The listing builds one solid part. Answer for the finished solid, in the listing's coordinates (mm). Give positions to 0.01 mm unless a question says otherwise; leave off trailing zeros. Write each loop counter-clockwise with the first axis right and the second up, starting at its lowest first coordinate (ties: lowest second). Pieces come first, ordered by that corner, then holes. Notation, with made-up numbers: M 81.5,69 L 100.5,69 A25 cw 100.5,108 Z; hole C 38,-37 d4. An arc over 180 degrees is marked long. Answer as a JSON object with one key per item and string values.
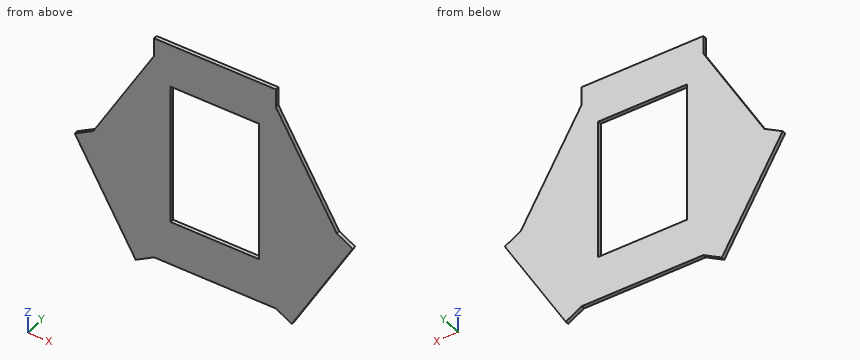
```python
from build123d import *

# Parameters (mm, degrees)
SKETCH1_W           = 120
SKETCH1_H           = 192
SKETCH1_W_2         = 165
SKETCH1_H_2         = 25
BOSS_EXTRUDE2_DEPTH = 5


with BuildPart() as part:
    # Sketch1 → Boss-Extrude2 (new body)
    with BuildSketch(Plane(origin=(0, 0, 0), x_dir=(1, 0, 0), z_dir=(0, 1, 0))):
        Polygon((-165, 0), (-82.5, -142.894191624), (82.5, -142.894191624), (165, 0), (82.5, 142.894191624), (-82.5, 142.894191624), align=None)
        with Locations((0, -13.105808376)):
            Rectangle(SKETCH1_W, SKETCH1_H, mode=Mode.SUBTRACT)
        Polygon((-82.5, 142.894191624), (-107.5, 157.327948354), (-190, 14.43375673), (-165, 0), align=None)
        Polygon((104.150635095, 155.394191624), (186.650635095, 12.5), (165, 0), (82.5, 142.894191624), align=None)
        with Locations((0, -155.394191624)):
            Rectangle(SKETCH1_W_2, SKETCH1_H_2)
    extrude(amount=BOSS_EXTRUDE2_DEPTH)


solid = part.part
```
1. A cutting plane is placed at B-B, the plane y = 3.45. Give the vertices of the cut face in (x, z), plus the area to 3 significant figures.
Verdict:
{"outline": "M -190,-14.43 L -107.5,-157.33 L -82.5,-142.89 L 82.5,-142.89 L 104.15,-155.39 L 186.65,-12.5 L 165,0 L 82.5,142.89 L 82.5,167.89 L -82.5,167.89 L -82.5,142.89 L -165,0 Z; hole M -60,-82.89 L 60,-82.89 L 60,109.11 L -60,109.11 Z", "area": "60,700 mm2"}
2. A cutting plane is placed at C-C, the plane z = 35. Give the vertices of the cut face in (x, y).
Verdict:
{"outline": "M -144.79,0 L -60,0 L -60,5 L -144.79,5 Z; M 60,0 L 144.79,0 L 144.79,5 L 60,5 Z"}
3. A cutting plane is placed at D-D, the plane x = -115.5. Give the vertices of the cut face in (y, z).
Verdict:
{"outline": "M 0,-143.47 L 5,-143.47 L 5,85.74 L 0,85.74 Z"}
4. Flat-ended cylindrical pins translate along their axes: pin 1 (1.5 mm diameter, centred on y = 2.5, z = 2, fed in from +X); pin 2 (1.5 mm diameter, centred on y = 2.5, z = 157, fed in from +X). Find the tip coordinate at first contact, or state that the pin passes through.
Verdict:
{"pin 1": "stops at x = 164.28", "pin 2": "stops at x = 82.5"}
5. A cutting plane is placed at A-A, the plane x = 39.5. Give the vertices of the cut face in (y, z), plus the area to 3 significant figures.
Verdict:
{"outline": "M 0,-142.89 L 5,-142.89 L 5,-82.89 L 0,-82.89 Z; M 0,109.11 L 5,109.11 L 5,167.89 L 0,167.89 Z", "area": "594 mm2"}
6. Consider line 1 along X through (y, z) = (0.6, 144.5); line 2 along X through (y, z) = (1.95, 21); line 3 along X through (y, z) = (4.35, 45.5). Determine where each line is inside the solid, lowest interval first.
Verdict:
{"line 1": "x = -82.5 to 82.5", "line 2": "x = -152.88 to -60, 60 to 152.88", "line 3": "x = -138.73 to -60, 60 to 138.73"}
